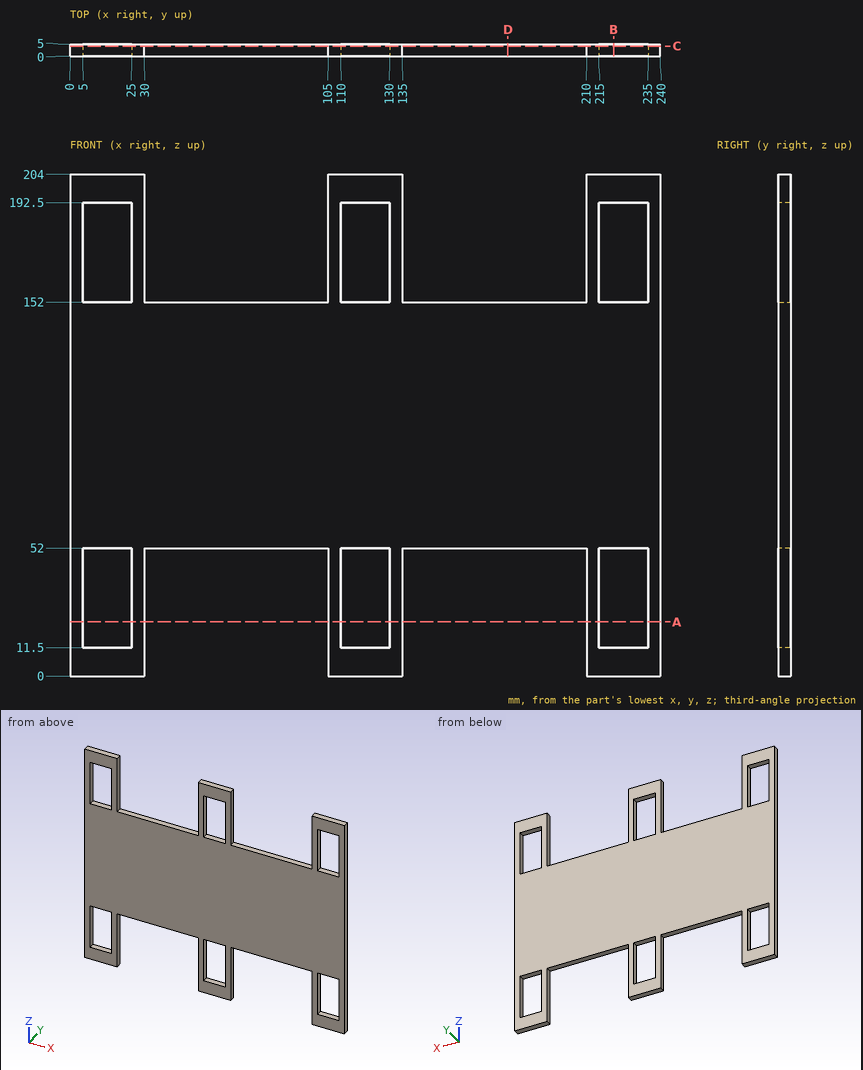
Design review of the part shown in the three views and the two pictorial views. Dimensions are in mm from the part's minimum x, y and z. Give positions to 0.01 mm unless a question says otherwise; leave off trailing zeros. Loops run counter-clockwise (first coordinate to the right, second up) from the corner with the lowest first, then second, coordinate; pieces in that order, holes last. Notation, with made-up numbers: (89, -34) -> (130, -34) arc R22 ccw to (130, -26) -> close; hole circle Ø5 at (77, -15.75). An arc over 180 degrees is marked (long way). Answer as a JSON object with one key per item and string values. Group by question number.
Q1. Take a section at D-D (x = 178). Write out the cut boundary in (y, z), plus the area to 3 significant figures.
Q2. Take a section at A-A (z = 22). Write out the cut boundary in (x, y), plus the area to 3 significant figures.
Q3. Wall thickness on line 1 along Z through (x, y) = (226, 2.2); line 2 along X through (y, z) = (3.7, 10); line 3 along X through (y, z) = (4.75, 176.5): over which ranges is each line inside the solid? List them lowest first.
Q4. Take a section at C-C (y = 4.1). State how many separate pieces and enclosed holes the cut face has, plus the area to 3 significant figures.
Q5. Take a section at B-B (x = 221). Write out the cut boundary in (y, z).
Answer below:
{
 "1": {"outline": "(0, 52) -> (5, 52) -> (5, 152) -> (0, 152) -> close", "area": "500 mm2"},
 "2": {"outline": "(0, 0) -> (5, 0) -> (5, 5) -> (0, 5) -> close; (25, 0) -> (30, 0) -> (30, 5) -> (25, 5) -> close; (105, 0) -> (110, 0) -> (110, 5) -> (105, 5) -> close; (130, 0) -> (135, 0) -> (135, 5) -> (130, 5) -> close; (210, 0) -> (215, 0) -> (215, 5) -> (210, 5) -> close; (235, 0) -> (240, 0) -> (240, 5) -> (235, 5) -> close", "area": "150 mm2"},
 "3": {"line 1": "z = 0 to 11.5, 52 to 152, 192.5 to 204", "line 2": "x = 0 to 30, 105 to 135, 210 to 240", "line 3": "x = 0 to 5, 25 to 30, 105 to 110, 130 to 135, 210 to 215, 235 to 240"},
 "4": {"separate pieces": "1", "enclosed holes": "6", "area": "28,500 mm2"},
 "5": {"outline": "(0, 0) -> (5, 0) -> (5, 11.5) -> (0, 11.5) -> close; (0, 52) -> (5, 52) -> (5, 152) -> (0, 152) -> close; (0, 192.5) -> (5, 192.5) -> (5, 204) -> (0, 204) -> close"}
}
